from build123d import *

# Parameters (mm, degrees)
SKETCH1_R               = 9.525
BOSS_EXTRUDE1_DEPTH     = 163.322
SKETCH2_OUTSIDE_W       = 54.156
SKETCH2_OUTSIDE_H       = 54.156
SKETCH2_OUTSIDE_R       = 8.128
CUT_EXTRUDE1_DEPTH      = 46.228
SKETCH3_OUTSIDE_W       = 54.156
SKETCH3_OUTSIDE_H       = 54.156
SKETCH3_OUTSIDE_R       = 6.223
CUT_EXTRUDE2_DEPTH      = 114.3
FILLET1_R               = 1.27
CUT_EXTRUDE3_DEPTH      = 10.525
CUT_EXTRUDE3_DEPTH_BACK = 10.525
FILLET2_R               = 0.762
FILLET3_R               = 0.762


with BuildPart() as part:
    # Sketch1 → Boss-Extrude1 (new body)
    with BuildSketch(Plane(origin=(0, 0, 0), x_dir=(1, 0, 0), z_dir=(0, 1, 0))):
        Circle(SKETCH1_R)
    extrude(amount=BOSS_EXTRUDE1_DEPTH)

    # Sketch2 outside → Cut-Extrude1 (cut)
    with BuildSketch(Plane(origin=(0, 0, 0), x_dir=(1, 0, 0), z_dir=(0, 1, 0))):
        Rectangle(SKETCH2_OUTSIDE_W, SKETCH2_OUTSIDE_H)
        Circle(SKETCH2_OUTSIDE_R, mode=Mode.SUBTRACT)
    extrude(amount=CUT_EXTRUDE1_DEPTH, mode=Mode.SUBTRACT)

    # Sketch3 outside → Cut-Extrude2 (cut)
    with BuildSketch(Plane(origin=(0, 163.322, 0), x_dir=(1, 0, 0), z_dir=(0, 1, 0))):
        Rectangle(SKETCH3_OUTSIDE_W, SKETCH3_OUTSIDE_H)
        Circle(SKETCH3_OUTSIDE_R, mode=Mode.SUBTRACT)
    extrude(amount=-CUT_EXTRUDE2_DEPTH, mode=Mode.SUBTRACT)

    # Fillet1
    fillet1_edges = [part.edges().sort_by_distance(p)[0] for p in [
        (-8.128, 46.228, 0),
    ]]
    fillet(fillet1_edges, radius=FILLET1_R)

    # Sketch4 → Cut-Extrude3 (cut, two sides)
    with BuildSketch(Plane.XY) as cut_extrude3_sk:
        with BuildLine():
            Line((2.63525, 125.222), (2.63525, 99.822))
            ThreePointArc((2.63525, 99.822), (0, 97.18675), (-2.63525, 99.822))
            Line((-2.63525, 99.822), (-2.63525, 125.222))
            ThreePointArc((-2.63525, 125.222), (0, 127.85725), (2.63525, 125.222))
        make_face()
    extrude(amount=CUT_EXTRUDE3_DEPTH, mode=Mode.SUBTRACT)
    extrude(cut_extrude3_sk.sketch, amount=-CUT_EXTRUDE3_DEPTH_BACK, mode=Mode.SUBTRACT)

    # Fillet2
    fillet2_edges = [part.edges().sort_by_distance(p)[0] for p in [
        (-6.223, 163.322, 0),
    ]]
    fillet(fillet2_edges, radius=FILLET2_R)

    # Fillet3
    fillet3_edges = [part.edges().sort_by_distance(p)[0] for p in [
        (-8.128, 0, 0),
    ]]
    fillet(fillet3_edges, radius=FILLET3_R)


solid = part.part
The model under review builds one solid part; all positions refer to its coordinate system, in mm. A direction names the side the tool comes from. Give positions to 0.01 mm unless a question says otherwise; leave off trailing zeros. Order: outer loops, then holes, each group sorted by start corner. A loop starts at its lowest first (then second) coordinate and runs counter-clockwise, first axis right, second up. Notation, with made-up numbers: M 50.5,33.25 L 104.5,33.25 A28 cw 104.5,72.25 Z; hole C -24.75,60 d3. An arc over 180 degrees is marked long. Use one line per item in the form item = value. Start each with the question number.
Item 1: Insertion check: pin 1 Ø3.5 at (y, z) = (117, -0.5) entering from +X; pin 2 Ø2 at (y, z) = (98, -2) entering from +X; pin 3 Ø1.5 at (x, y) = (-2.5, 52.5) entering from +Z. Each pin has a flat end and moves straight along its axis. Give the tip position at first contact, or say it passes through.
Item 2: For faces 4 (the cylindrical face through (-1.762, 22.551, 7.935)), 5 (the flat face through (0, 0, 0)), 6 (the cylindrical face through (5.75, 106.59, 2.38)), 7 (the flat face through (2.635, 113, 0)), list the 3-axis set-ups (+Z, -Z, +X, -X, +Y, -Y) from which the entire face can be reached by the end or side of a thin tool; tool diameter is ignored.
Item 3: We need section C-C on y = 109.5. Give the boundary of the cut face in (x, z).
Item 4: The part is to be moulded in two halves that separate along Y. For faces 1 (the flat face through (-2.635, 112, 0)), 2 (the cylindrical face through (-7.559, 47.605, 5.796)), 3 (the flat face through (6.2, 49.022, 2)), say which applies: pulls with the +Y half, pulls with the -Y half, needs draft (parallel to the pull), parting line crosses it, or undercut.
Item 5: We need section D-D on y = 88. Give the boundary of the cut face in (x, z), plus the area to 3 significant figures.
Item 6: To check wall thickness, follow line 1 along Z through (x, y) = (0, 52); line 2 along Y through (x, z) = (5.25, 5.25). State the ranges of each line that lie inside material, in increasing order. Write a range as from..to.
Item 7: We need section A-A on x = 0. Give the boundary of the cut face in (y, z) (3 decimals).
Completed:
q1.pin_1 = 6.22
q1.pin_2 = 6.14
q1.pin_3 = 5.97
q2.face_4 = -Y
q2.face_5 = +Z, -Z, +X, -X, -Y
q2.face_6 = +Y
q2.face_7 = +Z, -Z
q3.outline = M -2.64,-5.64 L -2.64,5.64 A6.22 ccw Z; M 2.64,-5.64 A6.22 ccw 2.64,5.64 Z
q4.face_1 = undercut
q4.face_2 = needs draft
q4.face_3 = pulls with the +Y half
q5.outline = C 0,0 d12.45
q5.area = 122 mm²
q6.line_1 = -6.22..6.22
q6.line_2 = 0..49.02
q7.outline = M 0,-7.366 A0.762 ccw 0.762,-8.128 L 44.958,-8.128 A1.27 cw 46.228,-9.398 L 46.228,-9.525 L 49.022,-9.525 L 49.022,-6.223 L 97.187,-6.223 L 97.187,6.223 L 49.022,6.223 L 49.022,9.525 L 46.228,9.525 L 46.228,9.398 A1.27 cw 44.958,8.128 L 0.762,8.128 A0.762 ccw 0,7.366 Z; M 127.857,-6.223 L 162.56,-6.223 A0.762 ccw 163.322,-5.461 L 163.322,5.461 A0.762 ccw 162.56,6.223 L 127.857,6.223 Z
